CAD build for the part. Positions are in the model's coordinates, mm. Face numbers are marked on the shaded views. Coordinates: 2 decimals unless noted, no trailing zeros. Loops run counter-clockwise (first coordinate to the right, second up) from the corner with the lowest first, then second, coordinate; pieces in that order, holes last. Notation, with made-up numbers: (36, 5.5) -> (59, 5.5) arc R12 ccw to (59, 25.5) -> close; hole circle Ø4 at (55, 73). An arc over 180 degrees is marked (long way). Return JSON: item names as keys, results as strings. Group by question number.
(1) Saw through at C-C on z = 26.5. Write the cut outline in (x, y), then the cut area to 3 significant figures.
(2) Saw through at A-A on z = 15.5. Write the cut outline in (x, y).
(3) Probe L1, parallel to Y at x = 10, z = 20; L2, parallel to Y at x = 26.5, z = 15; L3, parallel to Z at x = 49.5, y = 12. List the from-to ranges inside material, lowest first.
(4) Flat gauge pins, fed straight in: pin 1 Ø4 at (x, z) = (75.5, 8.5) entering from -Y; pin 2 Ø12 at (x, y) = (73.5, 20) entering from -Z; pin 3 Ø12 at (x, y) = (27.5, 18.5) entering from +Z. Where does each tip first touch, or does it go through?
(5) Saw through at B-B on y = -2. Write the cut outline in (x, z).
(6) Saw through at D-D on z = 20. Write the cut outline in (x, y), then the cut area to 3 significant figures.
(7) Mould opens along Z. For the marked faces 1, 2, 3 and 4 say: pulls with the +Z half, pulls with the -Z half, needs draft (parallel to the pull), parting line crosses it, or undercut.
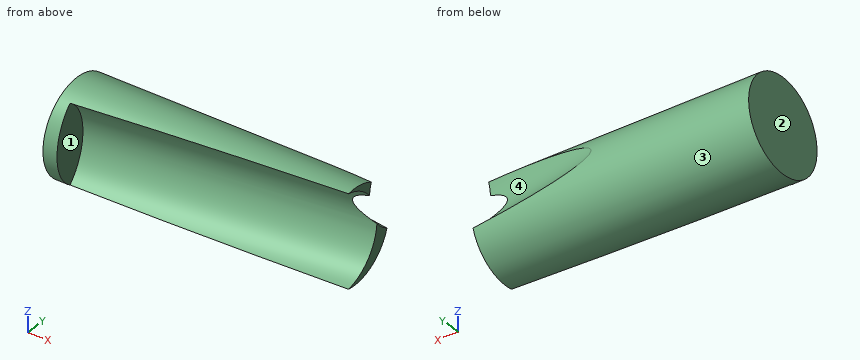
```python
from build123d import *

# Parameters (mm, degrees)
F0_R      = 15.707536
F1_DEPTH  = 92.8
F6_ANGLE  = -7.309847
F10_ANGLE = 11


with BuildPart() as f1:
    # F0 (on Right) → F1 (new body)
    with BuildSketch(Plane.YZ):
        with Locations((-37.135664, 18.661138)):
            Circle(F0_R)
    extrude(amount=F1_DEPTH)


with BuildPart() as f2_1:
    # F2: copy of F1
    add(f1.part.moved(Location((0, 47.6, 0))))


with BuildPart() as f3_1:
    # F3: copy of F2_1
    add(f2_1.part.moved(Location((0, 49.9, 0))))


with BuildPart() as f1_1:
    # F4: moved
    add(f1.part.moved(Location((4, 30.2, 0))))


with BuildPart() as f1_2:
    # F6: moved
    add(f1_1.part.rotate(Axis((0, 0, 16.515106), (0, 0, -1)), F6_ANGLE))


with BuildPart() as f3_1_1:
    # F7: moved
    add(f3_1.part.moved(Location((2.4, 0, 0))))


with BuildPart() as f3_1_2:
    # F8: moved
    add(f3_1_1.part.moved(Location((0, -10, 0))))


with BuildPart() as f3_1_3:
    # F9: moved
    add(f3_1_2.part.moved(Location((-0.2, 0, 8.6))))


with BuildPart() as f3_1_4:
    # F10: moved
    add(f3_1_3.part.rotate(Axis((0, 0, 16.515106), (0, 0, -1)), F10_ANGLE))


with BuildPart() as f2_1_1:
    add(f2_1.part)

    # F11: cut F1, F3_1
    add(f1_2.part, mode=Mode.SUBTRACT)
    add(f3_1_4.part, mode=Mode.SUBTRACT)


solid = f2_1_1.part
```
Geometry results:
{
 "1": {"outline": "(0, -3.15) -> (4.44, -3.15) -> (3.12, 7.13) -> (88.62, 18.1) -> (57.87, 24.08) -> (0, 24.08) -> close", "area": "980 mm²"},
 "2": {"outline": "(0, -4.92) -> (4.66, -4.92) -> (2.89, 8.89) -> (92.8, 20.42) -> (92.8, 22.66) -> (76.4, 25.85) -> (0, 25.85) -> close"},
 "3": {"L1": "10.07 to 26.11", "L2": "11.81 to 25.74", "L3": "3.03 to 9.2, 28.12 to 34.29"},
 "4": {"pin 1": "y = 12.7", "pin 2": "z = 3.36", "pin 3": "z = 34.24"},
 "5": {"outline": "(0, 9.1) -> (4.29, 9.1) -> (4.29, 28.22) -> (0, 28.22) -> close"},
 "6": {"outline": "(0, -5.19) -> (4.7, -5.19) -> (2.86, 9.15) -> (87.81, 20.05) -> (56.61, 26.11) -> (0, 26.11) -> close", "area": "986 mm²"},
 "7": {"face 1": "undercut", "face 2": "needs draft", "face 3": "parting line crosses it", "face 4": "undercut"}
}
